from build123d import *

# Parameters (mm, degrees)
F1_DEPTH  = 40
F3_DEPTH  = 37
F5_DEPTH  = 25
F6_R      = 5
F7_R      = 2
F9_W      = 5
F9_H      = 3.5
F9_H_2    = 3.4365921294
F10_DEPTH = 10
F11_W     = 20
F11_H     = 20.9946793665
F12_DEPTH = 2
F13_R     = 3.5
F14_DEPTH = 25


with BuildPart() as f1:
    # F0 (on Front) → F1 (new body)
    with BuildSketch(Plane.XZ):
        Polygon((-35.1044990334, 40.2309528088), (-35.0494137004, 1.2149916954), (54.9756615806, 8.540398173), (55.0351284044, 29.5349933202), align=None)
        Polygon((-49.999999976, 41.9984515125), (-49.999999976, -0.0015484875), (-35.0494137004, 1.2149916954), (-35.1044990334, 40.2309528088), align=None)
        Polygon((55.0351284044, 29.5349933202), (54.9756615806, 8.540398173), (59.9591903392, 8.9459115673), (59.9591903392, 18.9459115673), (60.0002953853, 28.9458270857), align=None)
    extrude(amount=F1_DEPTH)

    # F2 (on face) → F3 (cut)
    with BuildSketch(Plane.XZ.offset(40)):
        Polygon((-35.1044990334, 40.2309528088), (-35.0494137004, 1.2149916954), (54.9756615806, 8.540398173), (55.0351284044, 29.5349933202), align=None)
    extrude(amount=-F3_DEPTH, mode=Mode.SUBTRACT)

    # F4 (on face) → F5 (cut)
    with BuildSketch(Plane(origin=(-49.999999976, 0, 0), x_dir=(0, -1, 0), z_dir=(-1, 0, 0))):
        Polygon((3.5, 34.2484515125), (3.5, 20.9984515125), (3.5, 7.7484515125), (32.5, 7.7484515125), (32.5, 34.2484515125), align=None)
    extrude(amount=-F5_DEPTH, mode=Mode.SUBTRACT)

    # F6
    f6_edges = [f1.edges().sort_by_distance(p)[0] for p in [
        (-50, -20, 41.998452),
        (-50, -20, -0.001548),
        (-50, -40, 20.998452),
    ]]
    fillet(f6_edges, radius=F6_R)

    # F7
    f7_edges = [f1.edges().sort_by_distance(p)[0] for p in [
        (60.000295, -20, 28.945827),
        (59.95919, -20, 8.945912),
    ]]
    fillet(f7_edges, radius=F7_R)

    # F9 (on face) → F10 (cut)
    with BuildSketch(Plane(origin=(-35.0476284314, 0, -0.0494825765), x_dir=(0, 1, 0), z_dir=(0.9999990033, 0, 0.0014118652))):
        with Locations((-17.9936658144, 36.2820627093)):
            Rectangle(F9_W, F9_H)
        with Locations((-17.8817171156, 6.0796457964)):
            Rectangle(F9_W, F9_H_2)
    extrude(amount=-F10_DEPTH, mode=Mode.SUBTRACT)

    # F11 (on face) → F12 (cut)
    with BuildSketch(Plane(origin=(54.9510301824, 0, -0.1556478324), x_dir=(0, -1, 0), z_dir=(-0.9999959885, 0, 0.0028324712))):
        with Locations((18, 19.1934205725)):
            Rectangle(F11_W, F11_H)
    extrude(amount=-F12_DEPTH, mode=Mode.SUBTRACT)

    # F13 (on face) → F14 (cut)
    with BuildSketch(Plane(origin=(56.9510221594, 0, -0.1613127747), x_dir=(0, -1, 0), z_dir=(-0.9999959885, 0, 0.0028324712))):
        with Locations((18, 19.9799891561)):
            Circle(F13_R)
    extrude(amount=-F14_DEPTH, mode=Mode.SUBTRACT)


solid = f1.part
Can you work these out from the model? Positions are in its coordinate system, mm. A direction names the side the tool comes from. Round coordinates to 2 decimals unless told otherwise and drop trailing zeros. Order: outer loops, then holes, each group sorted by start corner. A loop starts at its lowest first (then second) coordinate and runs counter-clockwise, first axis right, second up. Notation, with made-up numbers: (75.5, 85) -> (86.5, 85) arc R10 ccw to (86.5, 94) -> close; hole circle Ø5 at (-3.75, 65). An arc over 180 degrees is marked (long way). Write each question's results on one line, items separated by ' | '. Start each with the question number.
Item 1: If we section it at A-A, the plane y = -26: Write out the boundary of the cut face in (x, z) (1 decimal).
Item 2: Will these pins go through, and if not, where does the flat tip stop? pin 1 (4 mm diameter, centred on y = -13.5, z = 13.5, fed in from +X); pin 2 (5 mm diameter, centred on x = 16, y = -6.5, fed in from +Z); pin 3 (11.5 mm diameter, centred on x = 2.5, z = 29.5, fed in from -Y); pin 4 (10 mm diameter, centred on y = -28.5, z = 36, fed in from +X).
Item 3: Which directions (+Z, -Z, +X, -X, +Y, -Y) give clear straight access to the entire face, cutting with the end or side of a thin tool? Please do faces 5 (the flat face through (-43, -21, 7.748)), 6 (the flat face through (9, -3, 21)), 7 (the cylindrical face through (59.4, -20.3, 9.4)).
Item 4: If we section it at D-D, the plane x = -39.5: Write out the boundary of the cut face in (y, z).
Item 5: If we section it at B-B, the plane z = 24.5: Write out the boundary of the cut face in (x, y).
Item 6: Thinking about a two-plate mould opening in Z: for faces 1 (the flat face through (-40, -20.382, 6)), 2 (the cylindrical face through (-48.431, -20.28, 1.785)), 3 (the flat face through (57, -40, 19)), 4 (the flat face through (-43, -3.5, 21)), which applies, +Z half, -Z half, draft (parallel to the pull), parting line (faces both ways), or undercut?
Item 7: If we section it at C-C, the plane y = -18: State how many separate pieces and enclosed holes the cut face has, then the cut area to 3 significant figures.
Item 8: Please list where these lines run through material, in increasing order: L1, parallel to Y at x = 48.5, z = 14; L2, parallel to X at y = -25, z = 22.5; L3, parallel to X at y = -29, z = 22.
Results:
1) outline: (-50, 5.4) arc R5 ccw to (-44.6, 0.4) -> (-35, 1.2) -> (-35.1, 7.7) -> (-50, 7.7) -> close; (-50, 34.2) -> (-35.1, 34.2) -> (-35.1, 40.2) -> (-44.4, 41.3) arc R5 ccw to (-50, 36.4) -> close; (57, 8.7) -> (58.1, 8.8) arc R2 ccw to (60, 10.8) -> (60, 18.9) -> (60, 27.2) arc R2 ccw to (58.2, 29.2) -> (57, 29.3) -> close
2) pin 1: stops at x = 59.96 | pin 2: passes through | pin 3: stops at y = -3 | pin 4: stops at x = -35.09
3) face 5: +X, -X | face 6: +Z, -Z, -Y | face 7: -Z, +X, +Y, -Y
4) outline: (-40, 0.85) -> (0, 0.85) -> (0, 40.75) -> (-40, 40.75) -> close; hole (-32.5, 7.75) -> (-3.5, 7.75) -> (-3.5, 34.25) -> (-32.5, 34.25) -> close; hole (-20.49, 34.48) -> (-15.49, 34.48) -> (-15.49, 37.98) -> (-20.49, 37.98) -> close; hole (-20.38, 4.31) -> (-15.38, 4.31) -> (-15.38, 7.74) -> (-20.38, 7.74) -> close
5) outline: (-50, -35) arc R5 ccw to (-45, -40) -> (-35.08, -40) -> (-35.08, -32.5) -> (-50, -32.5) -> close; (-50, -3.5) -> (-35.08, -3.5) -> (-35.08, -3) -> (55.02, -3) -> (55.02, -8) -> (57.02, -8) -> (57.02, -28) -> (55.02, -28) -> (55.02, -40) -> (59.98, -40) -> (59.98, 0) -> (-50, 0) -> close
6) face 1: undercut | face 2: -Z half | face 3: draft | face 4: undercut
7) separate pieces: 4 | enclosed holes: 0 | area: 164 mm2
8) L1: y = -3 to 0 | L2: x = 57.02 to 59.97 | L3: x = 55.01 to 59.97
